from build123d import *

# Parameters (mm, degrees)
SKETCH3_R           = 10
BOSS_EXTRUDE1_DEPTH = 15


with BuildPart() as part:
    # Sketch2 → Revolve1 (revolve)
    with BuildSketch(Plane.XY):
        Polygon((-120, 0), (120, 0), (120, 44.5), (-100, 44.5), (-100, 54.5), (-120, 54.5), align=None)
    revolve(axis=Axis((-120, 0, 0), (1, 0, 0)))

    # Sketch3 → Boss-Extrude1 (add)
    with BuildSketch(Plane.XY.offset(7.5)):
        with BuildLine():
            Line((120, 22.5), (155, 22.5))
            ThreePointArc((155, 22.5), (177.5, 0), (155, -22.5))
            Line((155, -22.5), (120, -22.5))
            Line((120, -22.5), (120, 22.5))
        make_face()
        with Locations((155, 0)):
            Circle(SKETCH3_R, mode=Mode.SUBTRACT)
    boss_extrude1 = extrude(amount=BOSS_EXTRUDE1_DEPTH)

    # Mirror1: Boss-Extrude1 across plane
    add(boss_extrude1.mirror(Plane.XY))


solid = part.part
CAD build for the part. Positions are in the model's coordinates, mm. A direction names the side the tool comes from. Round coordinates to 2 decimals unless told otherwise and drop trailing zeros. Write each loop counter-clockwise with the first axis right and the second up, starting at its lowest first coordinate (ties: lowest second). Pieces come first, ordered by that corner, then holes. Notation, with made-up numbers: M -17,48.25 L 10,48.25 A24 cw 10,63.25 Z; hole C -21.5,8.25 d3. An arc over 180 degrees is marked long. Put each result on its own line as item: value. Start each with the question number.
1) Drill centre lines: probe 1 along Y at (x, z) = (155, -13.25); probe 2 along Y at (x, z) = (-65.5, 1); probe 3 along X at (y, z) = (-47, 24). Where is each one in solid material? Low to high. Write a range as [from, to].
2) Saw through at B-B, the plane x = 127. Write the cut outline in (y, z), and give its area (3 significant figures).
3) Pull direction Y, two halves, no side cores. Call faces 6 (the cylindrical face through (164.237, -3.83, -14.895)), 7 (the cylindrical face through (164.237, -3.83, 14.895)), 8 (the flat face through (143, 0, -22.5)), 9 (the flat face through (138, -22.5, -15)): pulls with the +Y half, pulls with the -Y half, needs draft (parallel to the pull), parting line crosses it, or undercut.
4) Saw through at C-C, the plane z = 0. Write the cut outline in (x, y), and give its area (3 significant figures).
5) 3-axis set-ups, long thin cutter, end or side, ignore diameter. For faces 1 (the flat face through (138, -22.5, 15)), 2 (the flat face through (143, 0, 7.5)), 3 (the flat face through (-100, 45, 0)), 4 (the flat face through (143, 0, 22.5)), 5 (the flat face through (137, 22.5, -15)): which of +Z, -Z, +X, -X, +Y, -Y reach the whole face in a straight line?
6) Saw through at A-A, the plane y = 0. Write the cut outline in (x, z), and give its area (3 significant figures).
7) Saw through at D-D, the plane y = -38. Write the cut outline in (x, z).
8) Pin check, flat tips, straight feed: pin 1 Ø18 at (x, y) = (155, 0) entering from -Z; pin 2 Ø2 at (x, y) = (29.5, 9.5) entering from -Z; pin 3 Ø4.5 at (x, z) = (142, -12) entering from -Y; pin 4 Ø8 at (x, y) = (34, -23.5) entering from +Z. Stop position of each tip, or through.
Resolved:
1. probe 1: [-22.5, -10], [10, 22.5]
1. probe 2: [-44.49, 44.49]
1. probe 3: [-120, -100]
2. outline: M -22.5,-22.5 L 22.5,-22.5 L 22.5,-7.5 L -22.5,-7.5 Z; M -22.5,7.5 L 22.5,7.5 L 22.5,22.5 L -22.5,22.5 Z
2. area: 1,350 mm²
3. face 6: undercut
3. face 7: undercut
3. face 8: needs draft
3. face 9: pulls with the -Y half
4. outline: M -120,-54.5 L -100,-54.5 L -100,-44.5 L 120,-44.5 L 120,44.5 L -100,44.5 L -100,54.5 L -120,54.5 Z
4. area: 21,800 mm²
5. face 1: +Z, -Z, +X, -Y
5. face 2: +X, +Y, -Y
5. face 3: +X
5. face 4: +Z, +X, +Y, -Y
5. face 5: +Z, -Z, +X, +Y
6. outline: M -120,-54.5 L -100,-54.5 L -100,-44.5 L 120,-44.5 L 120,-22.5 L 145,-22.5 L 145,-7.5 L 120,-7.5 L 120,7.5 L 145,7.5 L 145,22.5 L 120,22.5 L 120,44.5 L -100,44.5 L -100,54.5 L -120,54.5 Z; M 165,-22.5 L 177.5,-22.5 L 177.5,-7.5 L 165,-7.5 Z; M 165,7.5 L 177.5,7.5 L 177.5,22.5 L 165,22.5 Z
6. area: 22,900 mm²
7. outline: M -120,-39.07 L -100,-39.07 L -100,-23.16 L 120,-23.16 L 120,23.16 L -100,23.16 L -100,39.07 L -120,39.07 Z
8. pin 1: through
8. pin 2: z = -43.68
8. pin 3: y = -22.5
8. pin 4: z = 40
